from build123d import *

# Parameters (mm, degrees)
BOSS_EXTRUDE2_DEPTH = 6.35


with BuildPart() as part:
    # Elevator Ball Support Rail → Boss-Extrude2 (new body)
    with BuildSketch(Plane(origin=(0, 0, 0), x_dir=(0, 0, -1), z_dir=(1, 0, 0))):
        with BuildLine():
            Line((63.5, 209.55), (63.5, 234.95))
            ThreePointArc((63.5, 234.95), (0.638207153, 208.911792847), (-25.4, 146.05))
            Line((-25.4, 146.05), (-25.4, -128.905))
            ThreePointArc((-25.4, -128.905), (-34.699359697, -151.355640303), (-57.15, -160.655))
            Line((-57.15, -160.655), (-57.15, -187.325))
            Line((-57.15, -187.325), (-50.8, -187.325))
            Line((-50.8, -187.325), (-50.8, -180.975))
            Line((-50.8, -180.975), (-46.609, -180.975))
            Line((-46.609, -180.975), (-46.609, -174.625))
            Line((-46.609, -174.625), (-48.649999982, -174.625))
            Line((-48.649999982, -174.625), (-48.649999982, -171.724999958))
            Line((-48.649999982, -171.724999958), (-46.609, -171.724999958))
            Line((-46.609, -171.724999958), (-46.609, -167.005))
            Line((-46.609, -167.005), (-42.291, -167.005))
            Line((-42.291, -167.005), (-42.291, -171.724999958))
            Line((-42.291, -171.724999958), (-40.250000018, -171.724999958))
            Line((-40.250000018, -171.724999958), (-40.250000018, -174.625))
            Line((-40.250000018, -174.625), (-42.291, -174.625))
            Line((-42.291, -174.625), (-42.291, -180.975))
            Line((-42.291, -180.975), (-38.1, -180.975))
            Line((-38.1, -180.975), (-38.1, -187.325))
            Line((-38.1, -187.325), (-31.75, -187.325))
            Line((-31.75, -187.325), (-31.75, -180.975))
            Line((-31.75, -180.975), (-18.788657666, -180.975))
            ThreePointArc((-18.788657666, -180.975), (-10.781328961, -196.174481473), (0, -209.55))
            Line((0, -209.55), (63.5, -209.55))
            ThreePointArc((63.5, -209.55), (18.598719395, -190.951280605), (0, -146.05))
            Line((0, -146.05), (0, 146.05))
            ThreePointArc((0, 146.05), (18.598719395, 190.951280605), (63.5, 209.55))
        make_face()
    extrude(amount=BOSS_EXTRUDE2_DEPTH)


solid = part.part
Read the model definition and answer for the solid it produces. Units are mm, in the model's axes. A direction names the side the tool comes from. Coordinates: 2 decimals unless noted, no trailing zeros. Write each loop counter-clockwise with the first axis right and the second up, starting at its lowest first coordinate (ties: lowest second). Pieces come first, ordered by that corner, then holes. Notation, with made-up numbers: (61.5, -5.5) -> (114.5, -5.5) arc R24 cw to (114.5, 32.5) -> close; hole circle Ø1 at (29, 48.5). An arc over 180 degrees is marked (long way). Return JSON: item names as keys, results as strings.
(1) Which of the six approach directions +Z, -Z, +X, -X, +Y, -Y give full straight-line access (tool end or side, diameter ignored) to faces 4 (the flat face through (0, 14, 11)), 5 (the cylindrical face through (3.131, -191.442, -19.095))?
Answers below:
{"face 4": "+Z, -Z, -X, +Y, -Y", "face 5": "-Z, +X, -X"}
(2) The part is cut by section C-C on y = 66. Give the vertices of the cut face in (x, z), then the cut area to 3 significant figures.
Answers below:
{"outline": "(0, 0) -> (6.35, 0) -> (6.35, 25.4) -> (0, 25.4) -> close", "area": "161 mm^2"}
(3) For a pull along Z with two mould halves and no side action, classify faces 1 (the flat face through (6.35, 14, 11)), 2 (the cylindrical face through (3.131, -151.107, 34.454)), 3 (the cylindrical face through (3.131, -195.973, 10.913)) as pulls with the +Z half, pulls with the -Z half, needs draft (parallel to the pull), parting line crosses it, or undercut.
Answers below:
{"face 1": "needs draft", "face 2": "pulls with the +Z half", "face 3": "undercut"}
(4) Each of these flat-tipped pins is pushed along its axis until it touches: P1, Ø1.5, axis at x = 1, z = -31, coming from the +Y side; P2, Ø1.9, axis at x = 1.5, y = -184.5, coming from the -Z side; P3, Ø3.5, axis at x = 3.5, z = 48.5, coming from the -Y side (3 decimals). Where does it stop, or does it pass through?
Answers below:
{"P1": "y = 229.09", "P2": "z = -13.7", "P3": "y = -180.975"}
(5) The part is cut by section D-D on y = 187. Give the vertices of the cut face in (x, z), then the cut area to 3 significant figures.
Answers below:
{"outline": "(0, -14.97) -> (6.35, -14.97) -> (6.35, 15.41) -> (0, 15.41) -> close", "area": "193 mm^2"}
(6) The part is cut by section A-A on z = -35. Give the vertices of the cut face in (x, y).
Answers below:
{"outline": "(0, -209.55) -> (6.35, -209.55) -> (6.35, -202.8) -> (0, -202.8) -> close; (0, 202.8) -> (6.35, 202.8) -> (6.35, 230.26) -> (0, 230.26) -> close"}
(7) Consider line 1 along Z through (x, y) = (0.75, -63.5); line 2 along Y through (x, z) = (1.5, 47.5) (3 decimals); line 3 along Y through (x, z) = (3, -40). Determine where each line is inside the solid, lowest interval first. Write a range as from..to.
Answers below:
{"line 1": "0..25.4", "line 2": "-180.975..-174.625, -171.725..-159.153", "line 3": "-209.55..-205.04, 205.04..231.79"}
